from build123d import *

# Parameters (mm, degrees)
PAD_DEPTH       = 40
SKETCH001_R     = 3.15
POCKET_DEPTH    = 8.001
POCKET001_DEPTH = 6
SKETCH003_R     = 5.75
POCKET002_DEPTH = 4
POCKET003_DEPTH = 4.501
FILLET_R        = 15
FILLET001_R     = 2
SKETCH005_R     = 1.6
POCKET004_DEPTH = 34.501
SKETCH006_W     = 8
SKETCH006_H     = 14.5
SKETCH006_H_2   = 10.5
PAD001_DEPTH    = 2
CHAMFER_SIZE    = 1.9


with BuildPart() as part:
    # Sketch → Pad (new body)
    with BuildSketch(Plane.XY):
        Polygon((-15, 0), (15, 0), (19.5, 0), (19.5, -30.2), (15, -30.2), (15, -8), (-15, -8), align=None)
    extrude(amount=PAD_DEPTH)

    # Sketch001 (on Face6 of Pad) → Pocket (cut, through all)
    with BuildSketch(Plane.XZ.offset(8)):
        with Locations((0, 15)):
            Circle(SKETCH001_R)
    extrude(amount=-POCKET_DEPTH, mode=Mode.SUBTRACT)

    # Sketch002 (on Face4 of Pocket) → Pocket001 (cut)
    with BuildSketch(Plane.XY.offset(40)):
        Polygon((-15, 0), (19.5, 0), (19.5, -10.6), (15, -10.6), (15, -8), (-15, -8), align=None)
    extrude(amount=-POCKET001_DEPTH, mode=Mode.SUBTRACT)

    # Sketch003 (on Face10 of Pocket001) → Pocket002 (cut)
    with BuildSketch(Plane.XZ.offset(8)):
        with Locations((0, 15)):
            Circle(SKETCH003_R)
    extrude(amount=-POCKET002_DEPTH, mode=Mode.SUBTRACT)

    # Sketch004 (on Face9 of Pocket002) → Pocket003 (cut, through all)
    with BuildSketch(Plane(origin=(15, 0, 0), x_dir=(0, -1, 0), z_dir=(-1, 0, 0))):
        with BuildLine():
            ThreePointArc((30.2, 10), (18.043042, 7.346447), (8, 0))
            Line((30.2, 0), (8, 0))
            Line((30.2, 10), (30.2, 0))
        make_face()
    extrude(amount=-POCKET003_DEPTH, mode=Mode.SUBTRACT)

    # Fillet
    fillet_edges = [part.edges().sort_by_distance(p)[0] for p in [
        (17.25, -30.2, 10),
    ]]
    fillet(fillet_edges, radius=FILLET_R)

    # Fillet001
    fillet001_edges = [part.edges().sort_by_distance(p)[0] for p in [
        (17.25, -10.6, 34),
    ]]
    fillet(fillet001_edges, radius=FILLET001_R)

    # Sketch005 (on Face10 of Fillet001) → Pocket004 (cut, through all)
    with BuildSketch(Plane.YZ.offset(19.5)):
        with Locations((-15.65, 37)):
            Circle(SKETCH005_R)
        with Locations((-25.15, 37)):
            Circle(SKETCH005_R)
    extrude(amount=-POCKET004_DEPTH, mode=Mode.SUBTRACT)

    # Sketch006 (on Face13 of Pocket004) → Pad001 (join)
    with BuildSketch(Plane(origin=(0, 0, 0), x_dir=(-1, 0, 0), z_dir=(0, 1, 0))):
        with Locations((0, 26.75)):
            Rectangle(SKETCH006_W, SKETCH006_H)
        with Locations((0, 5.25)):
            Rectangle(SKETCH006_W, SKETCH006_H_2)
    extrude(amount=PAD001_DEPTH)

    # Chamfer
    chamfer_edges = [part.edges().sort_by_distance(p)[0] for p in [
        (4, 2, 26.75),
        (4, 2, 5.25),
    ]]
    chamfer(chamfer_edges, length=CHAMFER_SIZE)


solid = part.part
Check sheet for the modelled part. Datum: model origin and axes. Units: mm. A direction names the side the tool comes from. Coordinates: 2 decimals unless noted, no trailing zeros. Loops run counter-clockwise (first coordinate to the right, second up) from the corner with the lowest first, then second, coordinate; pieces in that order, holes last. Notation, with made-up numbers: (50, -22.5) -> (100, -22.5) arc R18 cw to (100, -6.5) -> close; hole circle Ø10 at (7.25, 61). An arc over 180 degrees is marked (long way). Write item = value, one per line. Start each with the question number.
1. Depth check by flat-ended pin: P1, Ø1.2, axis at x = 16.5, z = 37.5, coming from the +Y side; P2, Ø10, axis at x = 2.5, z = 14.5, coming from the -Y side; P3, Ø1.6, axis at x = -1, y = 0.5, coming from the -Z side; P4, Ø2, axis at x = 1, y = 1, coming from the +Z side. Enter the tip coordinate at first touch or a pass-through.
2. Section check C-C on y = -26. Record the cut outline in (x, z), then the cut area to 3 significant figures.
3. Draft check along Z on faces 5 (the flat face through (2, -4, 34)), 6 (the flat face through (3, 1.1, 5.2)), 7 (the flat face through (-1, 1, 19.5)). Enter one of: released by +Z, released by -Z, zero draft, split by the parting line, or undercut.
4. Material ranges on line 1 (Z direction, x = 0, y = -5); line 2 (Z direction, x = 0, y = -1.05); line 3 (Y direction, x = -6, z = 18.5), recorded low to high.
5. Section check B-B on x = 17. Record the cut outline in (y, z), then the cut area to 3 significant figures.
6. Tool access check on faces 1 (the flat face through (-1, 1, 10.5)), 2 (the flat face through (17, -10.6, 38)), 3 (the flat face through (4, -8, 21)), 4 (the flat face through (-4, 1, 5)). Record the directions out of +Z, -Z, +X, -X, +Y, -Y that give a thin tool (end or side, any length) a straight path to the whole face; none if there is none.
7. Section check A-A on x = 0. Record the cut outline in (y, z).
8. Section check D-D on z = 27. Record the cut outline in (x, y), then the cut area to 3 significant figures.
Responses:
q1.P1 = -10.6
q1.P2 = -8
q1.P3 = 0
q1.P4 = 34
q2.outline = (15, 11.95) -> (19.5, 11.95) -> (19.5, 35.64) -> (15, 35.64) -> close; (15, 38.36) -> (19.5, 38.36) -> (19.5, 40) -> (15, 40) -> close
q2.area = 114 mm2
q3.face_5 = released by +Z
q3.face_6 = zero draft
q3.face_7 = undercut
q4.line_1 = 0 to 9.25, 20.75 to 34
q4.line_2 = 0 to 11.85, 18.15 to 34
q4.line_3 = -8 to 0
q5.outline = (-30.2, 22.36) arc R15 ccw to (-20.26, 8.24) arc R30.08 cw to (-8, 0) -> (0, 0) -> (0, 34) -> (-8.6, 34) arc R2 cw to (-10.6, 36) -> (-10.6, 40) -> (-30.2, 40) -> close; hole circle Ø3.2 at (-25.15, 37); hole circle Ø3.2 at (-15.65, 37)
q5.area = 950 mm2
q6.face_1 = +X, -X, +Y
q6.face_2 = +Z, +X, -X, +Y
q6.face_3 = +Z, -Z, -X, -Y
q6.face_4 = +Z, -Z, -X, +Y
q7.outline = (-8, 0) -> (2, 0) -> (2, 10.5) -> (0, 10.5) -> (0, 11.85) -> (-4, 11.85) -> (-4, 9.25) -> (-8, 9.25) -> close; (-8, 20.75) -> (-4, 20.75) -> (-4, 18.15) -> (0, 18.15) -> (0, 19.5) -> (2, 19.5) -> (2, 34) -> (-8, 34) -> close
q8.outline = (-15, -8) -> (15, -8) -> (15, -30.2) -> (19.5, -30.2) -> (19.5, 0) -> (4, 0) -> (4, 0.1) -> (2.1, 2) -> (-4, 2) -> (-4, 0) -> (-15, 0) -> close
q8.area = 390 mm2
